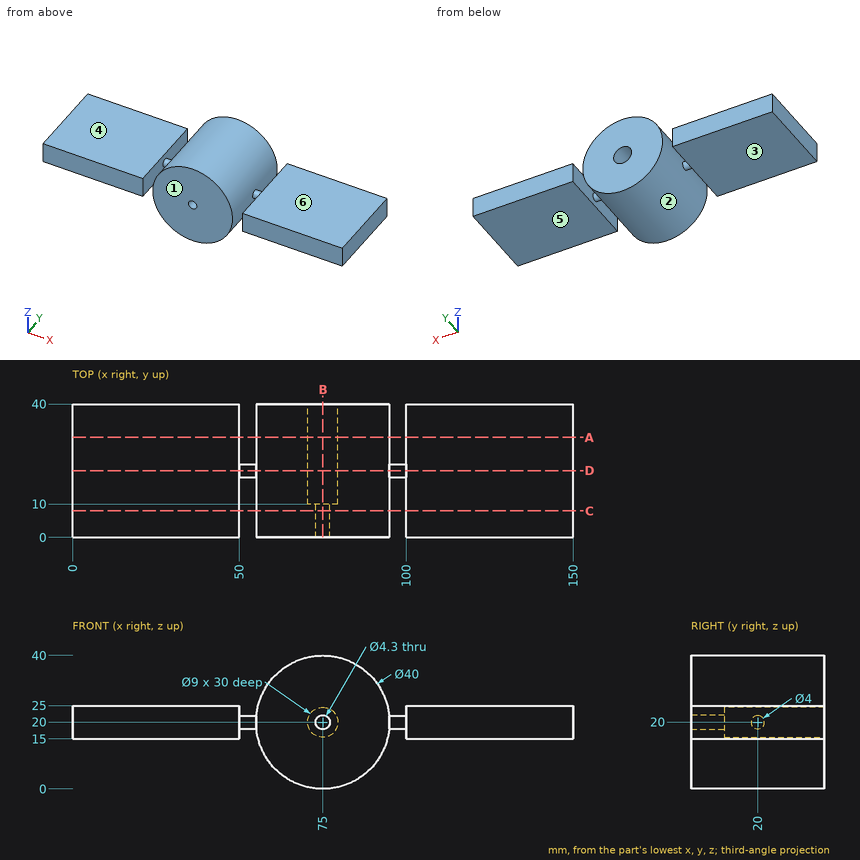
Answer from the drawing. Dimensions are ordinates in mm from the lowest x, y and z of the part. A direction names the side the tool comes from. Round coordinates to 2 decimals unless told otherwise and drop trailing zeros. Order: outer loops, then holes, each group sorted by start corner. A loop starts at its lowest first (then second) coordinate and runs counter-clockwise, first axis right, second up. Notation, with made-up numbers: (-22.5, 47) - (13.5, 47) arc R32 ccw to (13.5, 83) - close; hole circle Ø6 at (3, 7). An arc over 180 degrees is marked (long way). Put each result on its own line as item: value. Start each with the question number.
(1) Find section A-A (y = 30). Give the vertices of the cut face in (x, z).
(2) Determine the mould class of the marked faces 1 and 2 for opening direction X: released by +X, released by -X, zero draft, split by the parting line, or undercut.
(3) Straight lines are drawn through the part: probe 1 along X at (y, z) = (7, 20); probe 2 along Z at (x, y) = (37, 38.5); probe 3 along X at (y, z) = (22, 37.5). For each, find the intervals that lie inside material, in ascending order. Write a range as from..to.
(4) Find section D-D (y = 20). Give the vertices of the cut face in (x, z).
(5) Find section B-B (x = 75). Give the vertices of the cut face in (y, z), plus the area to 3 significant figures.
(6) For the marked faces 3, 4, 5 and 6, determine the directions among +Z, -Z, +X, -X, +Y, -Y from which every point of the face is accessible in a straight line to the end or side of a thin tool.
(7) Given P1, Ø5.5, axis at x = 75, z = 20, coming from the +Y side; P2, Ø2, axis at y = 11, z = 28, coming from the +X side (3 decimals); P3, Ø4, axis at y = 22.5, z = 34, coming from the -X side, each flat-ended and moving along its own axis, determine where each tip first touches the part or whether it passes through.
(8) Find section C-C (y = 8). Give the vertices of the cut face in (x, z).
Reply:
1. outline: (0, 15) - (50, 15) - (50, 25) - (0, 25) - close; circle Ø40 at (75, 20); (100, 15) - (150, 15) - (150, 25) - (100, 25) - close; hole circle Ø9 at (75, 20)
2. face 1: zero draft
2. face 2: undercut
3. probe 1: 0..50, 55..72.85, 77.15..95, 100..150
3. probe 2: 15..25
3. probe 3: 65.32..84.68
4. outline: (0, 15) - (50, 15) - (50, 18) - (55.1, 18) arc R20 ccw to (94.9, 18) - (100, 18) - (100, 15) - (150, 15) - (150, 25) - (100, 25) - (100, 22) - (94.9, 22) arc R20 ccw to (55.1, 22) - (50, 22) - (50, 25) - (0, 25) - close; hole circle Ø9 at (75, 20)
5. outline: (0, 0) - (40, 0) - (40, 15.5) - (10, 15.5) - (10, 17.85) - (0, 17.85) - close; (0, 22.15) - (10, 22.15) - (10, 24.5) - (40, 24.5) - (40, 40) - (0, 40) - close
5. area: 1,290 mm^2
6. face 3: -Z, -X, +Y, -Y
6. face 4: +Z, -X, +Y, -Y
6. face 5: -Z, +X, +Y, -Y
6. face 6: +Z, +X, +Y, -Y
7. P1: y = 10
7. P2: x = 93.735
7. P3: x = 59
8. outline: (0, 15) - (50, 15) - (50, 25) - (0, 25) - close; circle Ø40 at (75, 20); (100, 15) - (150, 15) - (150, 25) - (100, 25) - close; hole circle Ø4.3 at (75, 20)
